```python
from build123d import *

# Parameters (mm, degrees)
SKETCH1_W           = 30
SKETCH1_H           = 50
SKETCH1_R           = 4.25
BOSS_EXTRUDE1_DEPTH = 6
FILLET1_R           = 15
SKETCH2_R           = 20
CUT_EXTRUDE1_DEPTH  = 59.617403559


with BuildPart() as part:
    # Sketch1 → Boss-Extrude1 (new body)
    with BuildSketch(Plane(origin=(0, 0, 0), x_dir=(1, 0, 0), z_dir=(0, 1, 0))):
        with Locations((-15, 25)):
            Rectangle(SKETCH1_W, SKETCH1_H)
        with Locations(Location((-15, 35, 0), (0, 0, 270))):
            Circle(SKETCH1_R, mode=Mode.SUBTRACT)
    extrude(amount=BOSS_EXTRUDE1_DEPTH)

    # Fillet1
    fillet1_edges = [part.edges().sort_by_distance(p)[0] for p in [
        (-30, 3, -50),
        (0, 3, -50),
    ]]
    fillet(fillet1_edges, radius=FILLET1_R - 0.0001)  # a hair under: the kernel refuses the full size

    # Sketch2 → Cut-Extrude1 (cut, through all)
    with BuildSketch(Plane.ZY.offset(30)):
        with Locations((14.756354563, -7.5)):
            Circle(SKETCH2_R)
    extrude(amount=-CUT_EXTRUDE1_DEPTH, mode=Mode.SUBTRACT)


solid = part.part
```
The listing builds one solid part. Answer for the finished solid, in the listing's coordinates (mm). Coordinates: 2 decimals unless noted, no trailing zeros. Loops run counter-clockwise (first coordinate to the right, second up) from the corner with the lowest first, then second, coordinate; pieces in that order, holes last. Notation, with made-up numbers: (89.25, 89.25) -> (94.25, 89.25) arc R6 cw to (94.25, 100.25) -> close; hole circle Ø5 at (-27.75, 79.5). An arc over 180 degrees is marked (long way). Return JSON: item names as keys, results as strings. Group by question number.
(1) A cutting plane is placed at D-D on x = -4. Write down the section's boundary in (y, z).
(2) Determine the mould class of faces 1 (the flat face through (-15, 6, -25)), 2 (the cylindrical face through (-14.813, 2.958, -39.246)), 3 (the cylindrical face through (-25.72, 3.04, -45.49)), 4 (the flat face through (0, 3, -17)) for opening direction X: released by +X, released by -X, zero draft, split by the parting line, or undercut.
(3) Find the intervals of material crossed by probe 1 along X at (y, z) = (1.9, -35); probe 2 along X at (y, z) = (2.5, -38.5); probe 3 along Z at (x, y) = (-14, 1.25), in increasing order. Write a range as from..to.
(4) A cutting plane is placed at C-C on z = -32. Write down the section's boundary in (x, y), and give its area (3 significant figures).
(5) A cutting plane is placed at A-A on x = -11.5. Write down the section's boundary in (y, z), and give its area (3 significant figures).
(6) Given pin 1 Ø2 at (x, y) = (-8, 4) entering from -Z; pin 2 Ø7 at (x, z) = (-15, -35) entering from +Y; pin 3 Ø1.5 at (x, y) = (-18.5, 3.5) entering from -Z, each flat-ended and moving along its own axis, determine where each tip first touches the part or whether it passes through.
The answers:
{
 "1": {"outline": "(0, -45.2) -> (6, -45.2) -> (6, 0) arc R20 cw to (0, -3.78) -> close"},
 "2": {"face 1": "zero draft", "face 2": "undercut", "face 3": "released by -X", "face 4": "released by +X"},
 "3": {"probe 1": "x = -30..-19.25, -10.75..0", "probe 2": "x = -29.59..-17.41, -12.59..-0.41", "probe 3": "z = -49.97..-39.13, -30.87..-3.23"},
 "4": {"outline": "(-30, 0) -> (-18.01, 0) -> (-18.01, 6) -> (-30, 6) -> close; (-11.99, 0) -> (0, 0) -> (0, 6) -> (-11.99, 6) -> close", "area": "144 mm^2"},
 "5": {"outline": "(0, -49.59) -> (6, -49.59) -> (6, -37.41) -> (0, -37.41) -> close; (0, -32.59) -> (6, -32.59) -> (6, 0) arc R20 cw to (0, -3.78) -> close", "area": "256 mm^2"},
 "6": {"pin 1": "stops at z = -48.75", "pin 2": "passes through", "pin 3": "stops at z = -49.75"}
}
